Autodesk Inventor part; units mm, degrees
ref_plane "YZ Plane" through (0, 0, 0) normal (1, 0, 0) x (0, 1, 0)
ref_plane "XZ Plane" through (0, 0, 0) normal (0, 1, 0) x (-1, 0, 0)
ref_plane "XY Plane" through (0, 0, 0) normal (0, 0, 1) x (1, 0, 0)
sketch "Sketch1" plane through (0, 0, 0) normal (1, 0, 0) x (0, 1, 0)
  line L0 (0, 0) -> (331.78, 0)
  line L1 (331.78, 0) -> (331.78, -350)
  line L2 (331.78, -350) -> (0, -350)
  line L3 (0, -350) -> (0, 0)
  line L4 (239.261, -350) -> (331.78, -257.481)
  line L5 (120, -350) -> (115, -350)
  line L6 (115, -350) -> (115, -353)
  line L7 (115, -353) -> (120, -353)
  line L8 (120, -353) -> (120, -350)
  line L9 (115, -353) -> (130, -353)
  line L10 (130, -353) -> (130, -358)
  line L11 (130, -358) -> (115, -358)
  line L12 (115, -358) -> (115, -353)
  line L13 (90, -350) -> (95, -350)
  line L14 (95, -350) -> (95, -353)
  line L15 (95, -353) -> (90, -353)
  line L16 (90, -353) -> (90, -350)
  line L17 (90, -353) -> (105, -353)
  line L18 (105, -353) -> (105, -358)
  line L19 (105, -358) -> (90, -358)
  line L20 (90, -358) -> (90, -353)
  line L21 (60, -350) -> (65, -350)
  line L22 (65, -350) -> (65, -353)
  line L23 (65, -353) -> (60, -353)
  line L24 (60, -353) -> (60, -350)
  line L25 (60, -353) -> (75, -353)
  line L26 (75, -353) -> (75, -358)
  line L27 (75, -358) -> (60, -358)
  line L28 (60, -358) -> (60, -353)
  point P0 (117.5, -353)
  point P1 (115, -355.5)
  point P2 (130, -355.5)
  point P3 (95, -351.5)
  point P4 (90, -351.5)
  point P5 (90, -355.5)
  point P6 (60, -351.5)
  point P7 (65, -351.5)
  dimension "d0" = 350
  dimension "d1" = 331.78
  dimension "d2" = 239.261
  dimension "d3" = 45
  dimension "d27" = 3
  dimension "d28" = 5
  dimension "d29" = 5
  dimension "d30" = 15
  dimension "d31" = 115
  dimension "d32" = 5
  dimension "d33" = 15
  dimension "d34" = 5
  dimension "d35" = 25
  dimension "d36" = 15
  dimension "d37" = 5
  dimension "d38" = 65
extrude "Plate1" add sketch "Sketch1" along normal blind 2 contours L0 L1 L4 L2 L3 | L2 L22 L23 L24 | L23 L25 L26 L27 L28 | L8 L7 L6 L2 | L2 L14 L15 L16 | L9 L10 L11 L12 L7 | L15 L17 L18 L19 L20
sketch "Sketch2" plane through (0, 0, -2) normal (0, 0, 1) x (1, 0, 0)
  line L0 (0, 331.78) -> (0, 0)
  line L1 (0, 0) -> (200, 0)
  line L2 (200, 0) -> (200, 331.78)
  line L3 (200, 331.78) -> (0, 331.78)
edge flange "Flange1" height 200 angle 90 thickness 2 bend radius 2 thickness toward (0, 0, 1) relief tear relief width 2 relief depth 1 edges at (2, 165.89, 0) wall of the first edge with corners at (0, 331.78, -2) (0, 0, -2) (200, 0, -2) (200, 331.78, -2)
bend "Bend1"
corner "Corner1"
sketch "Sketch3" plane through (198, 0, 0) normal (1, 0, 0) x (0, 1, 0)
  line L0 (331.78, 0) -> (0, 0)
  line L1 (0, 0) -> (0, -350)
  line L2 (0, -350) -> (331.78, -350)
  line L3 (331.78, -350) -> (331.78, 0)
edge flange "Flange2" height 350 angle 90 thickness 2 bend radius 2 thickness toward (1, 0, 0) relief tear relief width 2 relief depth 1 edges at (200, 165.89, -2) wall of the first edge with corners at (198, 331.78, 0) (198, 0, 0) (198, 0, -350) (198, 331.78, -350)
bend "Bend2"
corner "Corner2"
sketch "Sketch4" plane through (200, 0, -350) normal (1, 0, 0) x (0, 0, -1)
  line L0 (-92.519, 331.78) -> (0, 239.261)
  line L1 (-346, 331.78) -> (0, 331.78)
  line L2 (0, 331.78) -> (0, 0)
  point P0 (-350, 0)
extrude "Cut1" cut sketch "Sketch4" against normal blind 2
sketch "Sketch5" plane through (200, 0, -4) normal (1, 0, 0) x (0, 0, -1)
  line L0 (0, 331.78) -> (0, 0)
  line L1 (346, 0) -> (0, 0)
  line L2 (346, 60) -> (346, 0)
  line L3 (354, 60) -> (346, 60)
  line L4 (354, 75) -> (354, 60)
  line L5 (349, 75) -> (354, 75)
  line L6 (349, 65) -> (349, 75)
  line L7 (346, 65) -> (349, 65)
  line L8 (346, 90) -> (346, 65)
  line L9 (354, 90) -> (346, 90)
  line L10 (354, 105) -> (354, 90)
  line L11 (349, 105) -> (354, 105)
  line L12 (349, 95) -> (349, 105)
  line L13 (346, 95) -> (349, 95)
  line L14 (346, 115) -> (346, 95)
  line L15 (354, 115) -> (346, 115)
  line L16 (354, 130) -> (354, 115)
  line L17 (349, 130) -> (354, 130)
  line L18 (349, 120) -> (349, 130)
  line L19 (346, 120) -> (349, 120)
  line L20 (346, 239.261) -> (346, 120)
  line L21 (253.481, 331.78) -> (346, 239.261)
  line L22 (0, 331.78) -> (253.481, 331.78)
  line L23 (346, 239.261) -> (253.481, 331.78)
  line L24 (0, 331.78) -> (253.481, 331.78)
  line L25 (0, 331.78) -> (0, 0)
  line L26 (346, 0) -> (0, 0)
  line L27 (346, 239.261) -> (346, 0)
  line L28 (346, 120) -> (354, 120)
  line L29 (354, 120) -> (354, 115)
  line L30 (354, 115) -> (346, 115)
  line L31 (346, 115) -> (346, 120)
  line L32 (354, 90) -> (346, 90)
  line L33 (346, 95) -> (354, 95)
  line L34 (354, 95) -> (354, 90)
  line L35 (354, 90) -> (346, 90)
  line L36 (346, 90) -> (346, 95)
  line L37 (346, 65) -> (354, 65)
  line L38 (354, 65) -> (354, 60)
  line L39 (354, 60) -> (346, 60)
  line L40 (346, 60) -> (346, 65)
  line L41 (354, 65) -> (349, 65)
  line L42 (349, 65) -> (349, 75)
  line L43 (349, 75) -> (354, 75)
  line L44 (354, 75) -> (354, 65)
  line L45 (354, 95) -> (349, 95)
  line L46 (349, 95) -> (349, 105)
  line L47 (349, 105) -> (354, 105)
  line L48 (354, 105) -> (354, 95)
  line L49 (354, 120) -> (349, 120)
  line L50 (349, 120) -> (349, 130)
  line L51 (349, 130) -> (354, 130)
  line L52 (354, 130) -> (354, 120)
  point P0 (-4, 0)
  point P1 (346, 65)
  point P2 (346, 60)
  point P3 (346, 95)
  point P4 (346, 90)
  point P5 (346, 120)
  point P6 (346, 115)
sheet face with bend "Face2" sketch "Sketch5" thickness 2 toward (-1, 0, 0) bend radius 2 contours L27 L7 L37 L4 L3 | L19 L28 L16 L15 L27 | L18 L17 L16 L28 | L37 L6 L5 L4 | L27 L13 L33 L10 L9 | L12 L11 L10 L33
bend "Bend3"
sketch "Sketch6" plane through (0, 0, 0) normal (-1, 0, 0) x (0, 0, 1)
  line L0 (-4, 0) -> (-4, 331.78)
  line L1 (-257.481, 331.78) -> (-4, 331.78)
  line L2 (-350, 239.261) -> (-257.481, 331.78)
  line L3 (-350, 120) -> (-350, 239.261)
  line L4 (-353, 120) -> (-350, 120)
  line L5 (-353, 130) -> (-353, 120)
  line L6 (-358, 130) -> (-353, 130)
  line L7 (-358, 115) -> (-358, 130)
  line L8 (-350, 115) -> (-358, 115)
  line L9 (-350, 95) -> (-350, 115)
  line L10 (-353, 95) -> (-350, 95)
  line L11 (-353, 105) -> (-353, 95)
  line L12 (-358, 105) -> (-353, 105)
  line L13 (-358, 90) -> (-358, 105)
  line L14 (-350, 90) -> (-358, 90)
  line L15 (-350, 65) -> (-350, 90)
  line L16 (-353, 65) -> (-350, 65)
  line L17 (-353, 75) -> (-353, 65)
  line L18 (-358, 75) -> (-353, 75)
  line L19 (-358, 60) -> (-358, 75)
  line L20 (-350, 60) -> (-358, 60)
  line L21 (-350, 0) -> (-350, 60)
  line L22 (-4, 0) -> (-350, 0)
  line L23 (-350, 60) -> (-350, 120)
  line L24 (-350, 120) -> (-353, 120)
  line L25 (-353, 130) -> (-358, 130)
  line L26 (-358, 60) -> (-350, 60)
  line L27 (-358, 60) -> (-358, 130)
  point P0 (0, 0)
extrude "Extrusion1" cut sketch "Sketch6" against normal through all contours L20 L19 L18 L17 L16 L23 | L23 L8 L7 L6 L5 L4 | L14 L13 L12 L11 L10 L23
equation "\"d33\" = d30"
equation "\"d36\" = d33"
equation "\"d25\" = Thickness"
equation "\"d4\" = Thickness"
equation "\"d5\" = BendReliefWidth"
equation "\"d6\" = BendReliefDepth"
equation "\"d7\" = MinimumRemnant"
equation "\"d8\" = TransitionRadius"
equation "\"d11\" = BendRadius"
equation "\"d12\" = CornerReliefSize"
equation "\"d13\" = GapSize"
equation "\"d14\" = JacobiRadiusSize"
equation "\"d15\" = BendReliefWidth"
equation "\"d16\" = BendReliefDepth"
equation "\"d17\" = MinimumRemnant"
equation "\"d18\" = TransitionRadius"
equation "\"d21\" = BendRadius"
equation "\"d22\" = CornerReliefSize"
equation "\"d23\" = GapSize"
equation "\"d24\" = JacobiRadiusSize"
equation "\"d39\" = BendRadius"
equation "\"d40\" = BendReliefWidth"
equation "\"d42\" = MinimumRemnant"
equation "\"d41\" = BendReliefDepth"
equation "\"d43\" = TransitionRadius"
equation "\"BendRadius\" = Thickness"
equation "\"BendReliefWidth\" = Thickness"
equation "\"BendReliefDepth\" = 0.5 * Thickness"
equation "\"CornerReliefSize\" = 4 * Thickness"
equation "\"MinimumRemnant\" = 2 * Thickness"
equation "\"TransitionRadius\" = BendRadius"
equation "\"JacobiRadiusSize\" = BendRadius"
equation "\"GapSize\" = Thickness"
properties part number "LzC-StoveCover" material "Steel"
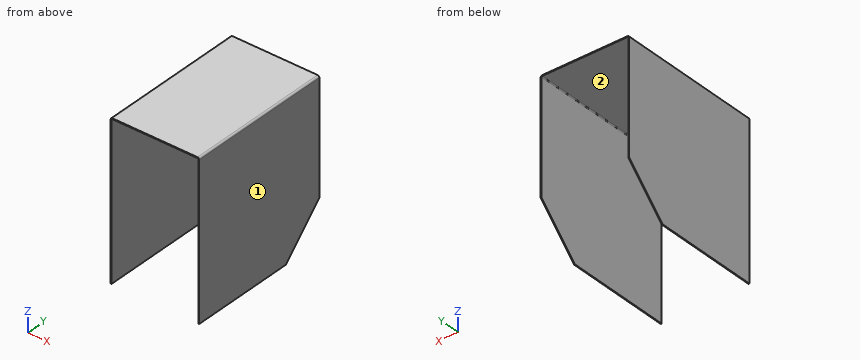
Here's how the part is built. I have some questions about the finished solid (model axes, mm). Face numbers are marked on the shaded views. A direction names the side the tool comes from. Coordinates: 2 decimals unless noted, no trailing zeros. Order: outer loops, then holes, each group sorted by start corner. A loop starts at its lowest first (then second) coordinate and runs counter-clockwise, first axis right, second up.
1) I need wall thicknesses on line 1 (X direction, y = 146.5, z = -251); line 2 (Z direction, x = 167.5, y = 157). Which ranges of each line are inside material? Lowest first, please.
2) Imagine slicing it at C-C on x = 111. List the corners of the cut face in (y, z) for me, and give its area (3 significant figures).
3) Imagine slicing it at A-A on z = -217. List the corners of the cut face in (x, y) for me, and give its area (3 significant figures).
4) Imagine slicing it at D-D on z = -315. List the corners of the cut face in (x, y) for me.
5) Will this pin go through, and if not, where does the flat tip stop? pin 1 (5 mm diameter, centred on x = 153.5, y = 193, fed in from -Z).
6) Which directions (+Z, -Z, +X, -X, +Y, -Y) give clear straight access to the entire face, cutting with the end or side of a thin tool? Please do the marked faces 1 and 2.
7) Imagine slicing it at B-B on y = 184.5. List the corners of the cut face in (x, z) for me.
Response values:
1. line 1: x = 0 to 2, 198 to 200
1. line 2: z = -2 to 0
2. outline: (0, -2) - (331.78, -2) - (331.78, 0) - (0, 0) - close
2. area: 664 mm2
3. outline: (0, 0) - (2, 0) - (2, 331.78) - (0, 331.78) - close; (198, 0) - (200, 0) - (200, 331.78) - (198, 331.78) - close
3. area: 1,330 mm2
4. outline: (0, 0) - (2, 0) - (2, 274.26) - (0, 274.26) - close; (198, 0) - (200, 0) - (200, 274.26) - (198, 274.26) - close
5. pin 1: stops at z = -2
6. face 1: +Z, -Z, +X, +Y, -Y
6. face 2: -Z, +Y, -Y
7. outline: (0, -350) - (2, -350) - (2, -4) arc R2 cw to (4, -2) - (196, -2) arc R2 cw to (198, -4) - (198, -350) - (200, -350) - (200, -4) arc R4 ccw to (196, 0) - (4, 0) arc R4 ccw to (0, -4) - close
